Autodesk Inventor part; units mm, degrees
ref_plane "YZ Plane" through (0, 0, 0) normal (1, 0, 0) x (0, 1, 0)
ref_plane "XZ Plane" through (0, 0, 0) normal (0, 1, 0) x (-1, 0, 0)
ref_plane "XY Plane" through (0, 0, 0) normal (0, 0, 1) x (1, 0, 0)
sketch "Sketch1" plane through (0, 0, 0) normal (0, 0, 1) x (1, 0, 0)
  line L0 (25, 25) -> (-25, 25)
  line L1 (-25, 25) -> (-25, -25)
  line L2 (-25, -25) -> (25, -25)
  line L3 (25, -25) -> (25, 25)
  line L4 (25, 25) -> (-25, -25) construction
  line L5 (-25, 25) -> (25, -25) construction
  point P0 (0, 0)
  dimension "d0" = 50
  dimension "d1" = 50
extrude "Extrusion1" add sketch "Sketch1" along normal blind 46.5
fillet "Fillet1" radius 5 4 edges at (-25, -25, 23.25) (25, -25, 23.25) (25, 25, 23.25) (-25, 25, 23.25)
sketch "Sketch2" plane through (0, 0, 46.5) normal (0, 0, 1) x (1, 0, 0)
  circle A0 centre (0, 0) radius 18
  dimension "d5" = 36
extrude "Extrusion2" add sketch "Sketch2" along normal blind 5
properties part number "Camera" material "Steel, Carbon"
Part model, mm, in its own coordinate system. A direction names the side the tool comes from. Coordinates: 2 decimals unless noted, no trailing zeros. Write each loop counter-clockwise with the first axis right and the second up, starting at its lowest first coordinate (ties: lowest second). Pieces come first, ordered by that corner, then holes. Notation, with made-up numbers: (53, 59.25) - (73, 59.25) arc R24 cw to (73, 69.25) - close; hole circle Ø5 at (86, 19). An arc over 180 degrees is marked (long way). Put each result on its own line as item: value.
1. Band-saw the part on A-A (x = 0). Write the cut outline in (y, z).
Final values:
outline: (-25, 0) - (25, 0) - (25, 46.5) - (18, 46.5) - (18, 51.5) - (-18, 51.5) - (-18, 46.5) - (-25, 46.5) - close
2. Band-saw the part on C-C (y = -21.5). Write the cut outline in (x, z), then the cut area to 3 significant figures.
Final values:
outline: (-24.77, 0) - (24.77, 0) - (24.77, 46.5) - (-24.77, 46.5) - close
area: 2,300 mm²
3. Probe line 1 along Z through (x, y) = (2.5, 20.5); line 2 along X through (y, z) = (21, 32.5); line 3 along X through (y, z) = (5.5, 47). List the from-to ranges inside material, lowest first. Write a range as [from, to].
Final values:
line 1: z = [0, 46.5]
line 2: x = [-24.9, 24.9]
line 3: x = [-17.14, 17.14]
4. 3-axis set-ups, long thin cutter, end or side, ignore diameter. For faces 1 (the flat face through (0, 0, 51.5)), 2 (the flat face through (-11, 17, 46.5)): which of +Z, -Z, +X, -X, +Y, -Y reach the whole face in a straight line?
Final values:
face 1: +Z, +X, -X, +Y, -Y
face 2: +Z
